from build123d import *

# Parameters (mm, degrees)
D10_PILOT_AND_M10X0P5_THREAD_ENVELOPE_START = -1
SKETCH1_R                                   = 5
SKETCH1_R_2                                 = 4
D10_PILOT_AND_M10X0P5_THREAD_ENVELOPE_DEPTH = 2.5
OUTER_RACE_INNER_SHOULDER_ID7P4_START       = 1.5
SKETCH2_R                                   = 5
SKETCH2_R_2                                 = 3.7
OUTER_RACE_INNER_SHOULDER_ID7P4_DEPTH       = 0.3
INBOARD_G10_RETENTION_FLANGE_H0P3_START     = 1.5
SKETCH3_R                                   = 7
SKETCH3_R_2                                 = 3.7
INBOARD_G10_RETENTION_FLANGE_H0P3_DEPTH     = 0.3
M14X0P5_BEARING_CAP_BOSS_START              = -1.6
SKETCH4_R                                   = 7
SKETCH4_R_2                                 = 4
M14X0P5_BEARING_CAP_BOSS_DEPTH              = 0.6
FLANGED_RACE_POCKET_D9P6_START              = -2.5
SKETCH5_R                                   = 7
SKETCH5_R_2                                 = 4.8
FLANGED_RACE_POCKET_D9P6_DEPTH              = 0.9
SKETCH6_R                                   = 0.6
TWO_PIN_WRENCH_HOLES_D1P2_DEPTH             = 0.301


with BuildPart() as part:
    # Sketch1 → D10_Pilot_And_M10x0p5_Thread_Envelope (new body)
    with BuildSketch(Plane.XY.offset(D10_PILOT_AND_M10X0P5_THREAD_ENVELOPE_START)):
        Circle(SKETCH1_R)
        Circle(SKETCH1_R_2, mode=Mode.SUBTRACT)
    extrude(amount=D10_PILOT_AND_M10X0P5_THREAD_ENVELOPE_DEPTH)

    # Sketch2 → Outer_Race_Inner_Shoulder_ID7p4 (add)
    with BuildSketch(Plane.XY.offset(OUTER_RACE_INNER_SHOULDER_ID7P4_START)):
        Circle(SKETCH2_R)
        Circle(SKETCH2_R_2, mode=Mode.SUBTRACT)
    extrude(amount=OUTER_RACE_INNER_SHOULDER_ID7P4_DEPTH)

    # Sketch3 → Inboard_G10_Retention_Flange_H0p3 (add)
    with BuildSketch(Plane.XY.offset(INBOARD_G10_RETENTION_FLANGE_H0P3_START)):
        Circle(SKETCH3_R)
        Circle(SKETCH3_R_2, mode=Mode.SUBTRACT)
    extrude(amount=INBOARD_G10_RETENTION_FLANGE_H0P3_DEPTH)

    # Sketch4 → M14x0p5_Bearing_Cap_Boss (add)
    with BuildSketch(Plane.XY.offset(M14X0P5_BEARING_CAP_BOSS_START)):
        Circle(SKETCH4_R)
        Circle(SKETCH4_R_2, mode=Mode.SUBTRACT)
    extrude(amount=M14X0P5_BEARING_CAP_BOSS_DEPTH)

    # Sketch5 → Flanged_Race_Pocket_D9p6 (add)
    with BuildSketch(Plane.XY.offset(FLANGED_RACE_POCKET_D9P6_START)):
        Circle(SKETCH5_R)
        Circle(SKETCH5_R_2, mode=Mode.SUBTRACT)
    extrude(amount=FLANGED_RACE_POCKET_D9P6_DEPTH)

    # Sketch6 → Two_Pin_Wrench_Holes_D1p2 (cut)
    with BuildSketch(Plane.XY.offset(1.8)):
        with Locations((-6, 0)):
            Circle(SKETCH6_R)
        with Locations((6, 0)):
            Circle(SKETCH6_R)
    extrude(amount=-TWO_PIN_WRENCH_HOLES_D1P2_DEPTH, mode=Mode.SUBTRACT)


solid = part.part
Geometry: final body of the model. Coordinates: model frame, mm. A direction names the side the tool comes from. Round coordinates to 2 decimals unless told otherwise and drop trailing zeros. Loops run counter-clockwise (first coordinate to the right, second up) from the corner with the lowest first, then second, coordinate; pieces in that order, holes last. Notation, with made-up numbers: M 83.5,74.25 L 99.5,74.25 A21 cw 99.5,97.25 Z; hole C -9,-14.75 d10. An arc over 180 degrees is marked long. Put each result on its own line as item: value. Start each with the question number.
(1) Section query B-B (x = 0). Return loops of the section in (y, z), then the cut area to 3 significant figures.
(2) Set-up query: faces 4 (the face through (2.58, 4.05, -2.06)), 5 (the face through (-1.08, -4.88, 0.23)), 6 (the face through (3, -3, 1.8)), 7 (the face through (-5.72, -0.53, 1.65)). Return all of +Z, -Z, +X, -X, +Y, -Y with unobstructed straight access to the full face (end or side cutting, diameter ignored); none if empty.
(3) Draft query along Z for faces 1 (the face through (-2, 4, -1.6)), 2 (the face through (-0.867, -3.905, -0.072)), 3 (the face through (-2, 5, -1)). Return one class per face: +Z half, -Z half, draft (parallel to the pull), parting line (faces both ways), or undercut.
(4) Section query A-A (y = 0). State how many separate pieces and enclosed holes the cut face has, then the cut area to 3 significant figures.
(5) Section query D-D (x = -5.75). Return loops of the section in (y, z), then the cut area to 3 significant figures.
(6) Contact query for flat-ended pins moving along their axis: pin 1 Ø1 at (y, z) = (-1.5, -1.5) entering from +X; pin 2 Ø1 at (x, y) = (-6, 0) entering from +Z; pin 3 Ø7.5 at (x, y) = (-1.5, 0) entering from -Z; pin 4 Ø1.5 at (y, z) = (1, -1.5) entering from +X. Output: stop coordinate, or through.
(7) Section query C-C (y = -1.5). Return loops of the section in (x, z), then the cut area to 3 significant figures.
(8) Material intervals for line 1 along Y through (x, z) = (0, -0.1); line 2 along Z through (x, y) = (-3.25, 4.5); line 3 along Z through (x, y) = (3.5, 3), sorted ascending. Write a range as [from, to].
Findings below:
1. outline: M -7,-2.5 L -4.8,-2.5 L -4.8,-1.6 L -4,-1.6 L -4,1.5 L -3.7,1.5 L -3.7,1.8 L -7,1.8 L -7,1.5 L -5,1.5 L -5,-1 L -7,-1 Z; M 3.7,1.5 L 4,1.5 L 4,-1.6 L 4.8,-1.6 L 4.8,-2.5 L 7,-2.5 L 7,-1 L 5,-1 L 5,1.5 L 7,1.5 L 7,1.8 L 3.7,1.8 Z
1. area: 14.5 mm2
2. face 4: -Z
2. face 5: none
2. face 6: +Z, +X, -X, +Y, -Y
2. face 7: +Z
3. face 1: -Z half
3. face 2: draft
3. face 3: undercut
4. separate pieces: 4
4. enclosed holes: 0
4. area: 13.8 mm2
5. outline: M -3.99,-2.5 L 3.99,-2.5 L 3.99,-1 L -3.99,-1 Z; M -3.99,1.5 L -0.55,1.5 L -0.55,1.8 L -3.99,1.8 Z; M 0.55,1.5 L 3.99,1.5 L 3.99,1.8 L 0.55,1.8 Z
5. area: 14.0 mm2
6. pin 1: stops at x = 6.93
6. pin 2: stops at z = -1
6. pin 3: stops at z = -2.5
6. pin 4: stops at x = 7
7. outline: M -6.84,-2.5 L -4.56,-2.5 L -4.56,-1.6 L -3.71,-1.6 L -3.71,1.5 L -3.38,1.5 L -3.38,1.8 L -6.84,1.8 L -6.84,1.5 L -4.77,1.5 L -4.77,-1 L -6.84,-1 Z; M 3.38,1.5 L 3.71,1.5 L 3.71,-1.6 L 4.56,-1.6 L 4.56,-2.5 L 6.84,-2.5 L 6.84,-1 L 4.77,-1 L 4.77,1.5 L 6.84,1.5 L 6.84,1.8 L 3.38,1.8 Z
7. area: 15.2 mm2
8. line 1: y = [-5, -4], [4, 5]
8. line 2: z = [-2.5, -1], [1.5, 1.8]
8. line 3: z = [-1.6, 1.8]
